Can you work these out from the drawing? Everything is in mm from the part's minimum corner. Give positions to 0.01 mm unless a question says otherwise; leave off trailing zeros. Write each loop counter-clockwise with the first axis right and the second up, starting at its lowest first coordinate (ties: lowest second). Pieces come first, ordered by that corner, then holes. Notation, with made-up numbers: (81.25, 49.5) -> (120.25, 49.5) arc R25 ccw to (120.25, 83.5) -> close; hole circle Ø3 at (84, -8.75). An arc over 180 degrees is marked (long way). Write item = value, one per line. Start each with the question number.
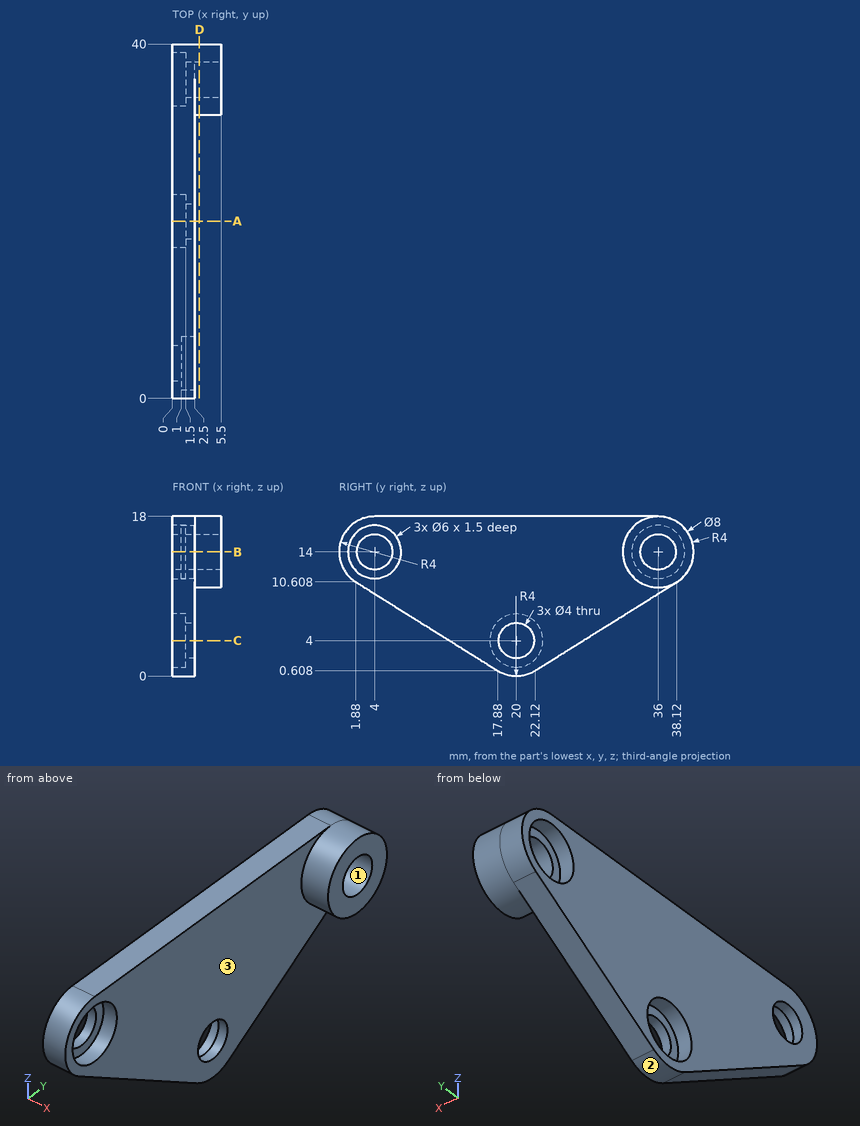
(1) Imagine slicing it at A-A (y = 20). Please give me the cut outline in (x, z), then the cut area to 3 significant figures.
(2) We'd pull the mould along Y, two halves only. Please class the marked faces 1, 2 and 3: released by +Y, released by -Y, zero draft, split by the parting line, or undercut.
(3) If I drill on line 1 along Y through (x, z) = (2.15, 14); line 2 along Y through (x, z) = (1.1, 14); line 3 along Y through (x, z) = (3.7, 14), over which ranges is the centre line in solid material (lowest first)? Write a range as from..to.
(4) Imagine slicing it at B-B (z = 14). Please give me the cut outline in (x, y).
(5) Imagine slicing it at C-C (z = 4). Please give me the cut outline in (x, y), then the cut area to 3 significant figures.
(6) Imagine slicing it at D-D (x = 3.05). Please give me the cut outline in (y, z).
(7) I'm going to push flat-ended pins straight in: pin 1 (10 mm diameter, centred on y = 8, z = 3.5, fed in from +X); pin 2 (4.5 mm diameter, centred on y = 20, z = 4, fed in from -X); pin 3 (1 mm diameter, centred on x = 3.5, z = 14, fed in from -Y). Where does each tip first touch, or does it pass through?
Answers below:
q1.outline = (0, 0) -> (2.5, 0) -> (2.5, 2) -> (1.5, 2) -> (1.5, 1) -> (0, 1) -> close; (0, 7) -> (1.5, 7) -> (1.5, 6) -> (2.5, 6) -> (2.5, 18) -> (0, 18) -> close
q1.area = 32.0 mm^2
q2.face_1 = undercut
q2.face_2 = split by the parting line
q2.face_3 = zero draft
q3.line_1 = 0..1, 7..34, 38..40
q3.line_2 = 0..1, 7..33, 39..40
q3.line_3 = 32..34, 38..40
q4.outline = (0, 0) -> (2.5, 0) -> (2.5, 1) -> (1, 1) -> (1, 2) -> (0, 2) -> close; (0, 6) -> (1, 6) -> (1, 7) -> (2.5, 7) -> (2.5, 32) -> (5.5, 32) -> (5.5, 34) -> (1.5, 34) -> (1.5, 33) -> (0, 33) -> close; (0, 39) -> (1.5, 39) -> (1.5, 38) -> (5.5, 38) -> (5.5, 40) -> (0, 40) -> close
q5.outline = (0, 12.45) -> (2.5, 12.45) -> (2.5, 18) -> (1.5, 18) -> (1.5, 17) -> (0, 17) -> close; (0, 23) -> (1.5, 23) -> (1.5, 22) -> (2.5, 22) -> (2.5, 27.55) -> (0, 27.55) -> close
q5.area = 24.7 mm^2
q6.outline = circle Ø8 at (36, 14); hole circle Ø4 at (36, 14)
q7.pin_1 = 2.5
q7.pin_2 = 1.5
q7.pin_3 = 32
